The figure shows three views and two pictorial views of one solid part (mm, origin at its lowest corner). Answer the questions. Coordinates: 2 decimals unless noted, no trailing zeros. Order: outer loops, then holes, each group sorted by start corner. A loop starts at its lowest first (then second) coordinate and runs counter-clockwise, first axis right, second up.
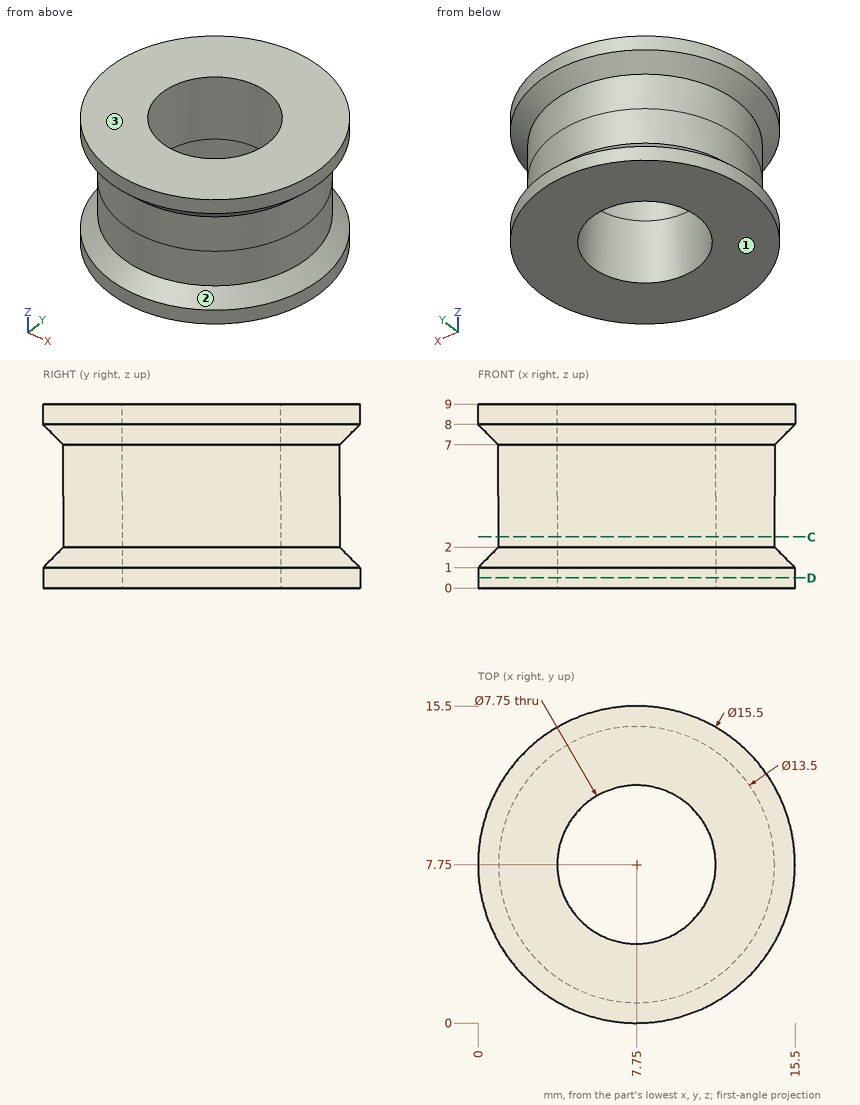
Q1. Each of these flat-tipped pins is pushed along its axis until it touches: P1, Ø5, axis at y = 13, z = 7.5, coming from the +X side; P2, Ø4.5, axis at x = 7.5, y = 10.5, coming from the +Z side; P3, Ø2, axis at y = 2.5, z = 2, coming from the +X side (1 decimal); P4, Ø2, axis at x = 3.5, z = 7.5, coming from the -Y side. Where does it stop, or does it pass through?
Q2. The part is cut by section D-D, the plane z = 0.5. Determine the outline of the cut face in (x, y) (3 decimals), then the cut area to 4 significant figures.
Q3. The part is cut by section C-C, the plane z = 2.5. Determine the outline of the cut face in (x, y) (3 decimals).
Q4. Straight lines are drawn through the part: L1, parallel to Y at x = 7.75, z = 6.3 (3 decimals); L2, parallel to Z at x = 12.25, y = 13.5; L3, parallel to Y at x = 7.75, z = 1.5 (1 decimal). For each, find the intervals that lie inside material, in ascending order.
Q5. Determine the mould class of the marked faces 1, 2 and 3 for opening direction Z: +Z half, -Z half, draft (parallel to the pull), parting line (faces both ways), or undercut.
Computed values:
1. P1: stops at x = 14.98
1. P2: stops at z = 9
1. P3: stops at x = 13.7
1. P4: stops at y = 0.78
2. outline: circle Ø15.5 at (7.75, 7.75); hole circle Ø7.75 at (7.75, 7.75)
2. area: 141.5 mm2
3. outline: circle Ø13.5 at (7.75, 7.75); hole circle Ø7.75 at (7.75, 7.75)
4. L1: y = 1 to 3.875, 11.625 to 14.5
4. L2: z = 0 to 1.45, 7.55 to 9
4. L3: y = 0.5 to 3.9, 11.6 to 15
5. face 1: -Z half
5. face 2: undercut
5. face 3: +Z half
